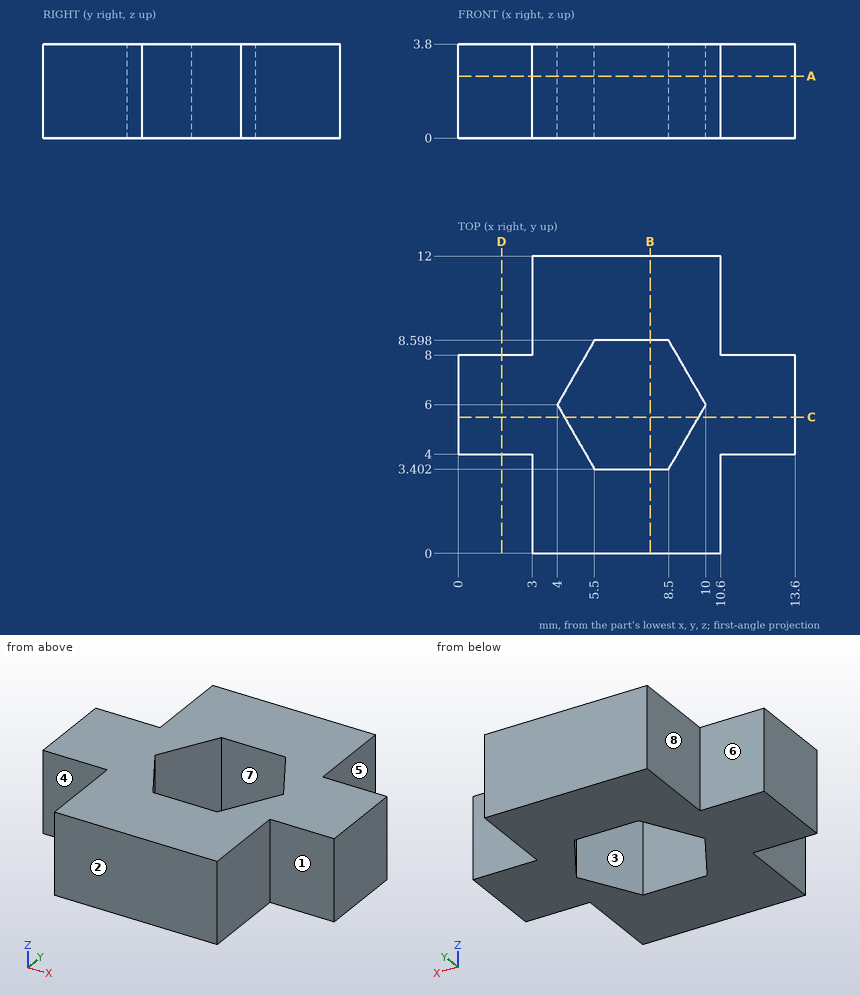
Could you check a few things on this drawing? It's one solid part, dimensions in mm from its lowest x, y, z. A direction names the side the tool comes from. Coordinates: 2 decimals unless noted, no trailing zeros. Order: outer loops, then holes, each group sorted by start corner. A loop starts at its lowest first (then second) coordinate and runs counter-clockwise, first axis right, second up.
1. If we section it at D-D (x = 1.75): Please give me the cut outline in (y, z).
2. For the marked faces 1, 2, 3, 4 and 5, which set-ups out of +Z, -Z, +X, -X, +Y, -Y let a thin tool reach every point of the face, with its end or its side?
3. If we section it at C-C (y = 5.5): Please give me the cut outline in (x, z), then the cut area to 3 significant figures.
4. Thinking about a two-plate mould opening in X: for the marked faces 6, 7 and 8, which applies, +X half, -X half, draft (parallel to the pull), parting line (faces both ways), or undercut?
5. I need wall thicknesses on line 1 (Y direction, x = 8, z = 0.8); line 2 (Y direction, x = 1.5, z = 0.4); line 3 (X direction, y = 10.25, z = 1.4). Which ranges of each line are inside material? Lowest first, please.
6. If we section it at B-B (x = 7.75): Please give me the cut outline in (y, z).
7. I'm going to push flat-ended pins straight in: pin 1 (1.9 mm diameter, centred on y = 2.5, z = 2, fed in from -X); pin 2 (0.9 mm diameter, centred on x = 1.5, z = 1.5, fed in from +Y); pin 3 (1.9 mm diameter, centred on y = 1.5, z = 2, fed in from +X). Where does each tip first touch, or does it pass through?
8. If we section it at A-A (z = 2.5): Please give me the cut outline in (x, y), then the cut area to 3 significant figures.
Entries:
1. outline: (4, 0) - (8, 0) - (8, 3.8) - (4, 3.8) - close
2. face 1: +Z, -Z, +X, -Y
2. face 2: +Z, -Z, +X, -X, -Y
2. face 3: +Z, -Z
2. face 4: +Z, -Z, -X, -Y
2. face 5: +Z, -Z, +X, +Y
3. outline: (0, 0) - (4.29, 0) - (4.29, 3.8) - (0, 3.8) - close; (9.71, 0) - (13.6, 0) - (13.6, 3.8) - (9.71, 3.8) - close
3. area: 31.1 mm2
4. face 6: draft
4. face 7: undercut
4. face 8: -X half
5. line 1: y = 0 to 3.4, 8.6 to 12
5. line 2: y = 4 to 8
5. line 3: x = 3 to 10.6
6. outline: (0, 0) - (3.4, 0) - (3.4, 3.8) - (0, 3.8) - close; (8.6, 0) - (12, 0) - (12, 3.8) - (8.6, 3.8) - close
7. pin 1: stops at x = 3
7. pin 2: stops at y = 8
7. pin 3: stops at x = 10.6
8. outline: (0, 4) - (3, 4) - (3, 0) - (10.6, 0) - (10.6, 4) - (13.6, 4) - (13.6, 8) - (10.6, 8) - (10.6, 12) - (3, 12) - (3, 8) - (0, 8) - close; hole (4, 6) - (5.5, 3.4) - (8.5, 3.4) - (10, 6) - (8.5, 8.6) - (5.5, 8.6) - close
8. area: 91.8 mm2
